Part model, mm, in its own coordinate system. Face numbers are marked on the shaded views. Coordinates: 2 decimals unless noted, no trailing zeros. Loops run counter-clockwise (first coordinate to the right, second up) from the corner with the lowest first, then second, coordinate; pieces in that order, holes last. Notation, with made-up numbers: M 70,-31.75 L 78,-31.75 A28 cw 78,-6.75 Z; hole C 33.5,61 d8. An arc over 180 degrees is marked long. Answer as a JSON object with one key per item and string values. Group by question number.
1. Drill centre lines: L1, parallel to X at y = 0, z = 7.2; L2, parallel to Y at x = 0, z = 2.1 (3 decimals); L3, parallel to X at y = -5, z = 10.5 (3 decimals). Where is each one in solid material? Low to high.
2. Drop a flat-ended pin along its axis: pin 1 Ø7.5 at (x, y) = (0, 0) entering from +Z. Give the stop position or say it passes through.
3. Mould opens along Y. For the marked faces 1, 2 and 3 say: released by +Y, released by -Y, zero draft, split by the parting line, or undercut.
4. Saw through at D-D on z = 2.25. Write the cut outline in (x, y) (3 decimals), then the cut area to 3 significant figures.
5. Saw through at C-C on z = 12. Write the cut outline in (x, y).
6. Saw through at B-B on x = 0. Write the cut outline in (y, z) (3 decimals), then the cut area to 3 significant figures.
7. Saw through at A-A on y = 0. Write the cut outline in (x, z) (3 decimals), then the cut area to 3 significant figures.
from build123d import *

# Parameters (mm, degrees)
F2_DEPTH = 25.4


with BuildPart() as f2:
    # F0 (on Front) → F2 (new body, symmetric)
    with BuildSketch(Plane.XZ):
        with BuildLine():
            Line((-19.05, 17.7), (-19.05, 0))
            Line((-19.05, 0), (19.05, 0))
            Line((19.05, 0), (19.05, 17.7))
            Line((19.05, 17.7), (12.541531, 17.7))
            ThreePointArc((12.541531, 17.7), (0, 7), (-12.541531, 17.7))
            Line((-12.541531, 17.7), (-19.05, 17.7))
        make_face()
    extrude(amount=F2_DEPTH, both=True)

    # F1 (on Front) → F3 (revolve, cut)
    with BuildSketch(Plane.XZ):
        Polygon((0, 17.176644), (-6.3, 17.176644), (-6.3, 7), (-6.3, 6.479864), (-3.275, 3), (-3.275, 0), (0, 0), align=None)
    revolve(axis=Axis((0, 0, 8.588322), (0, 0, -1)), mode=Mode.SUBTRACT)


solid = f2.part
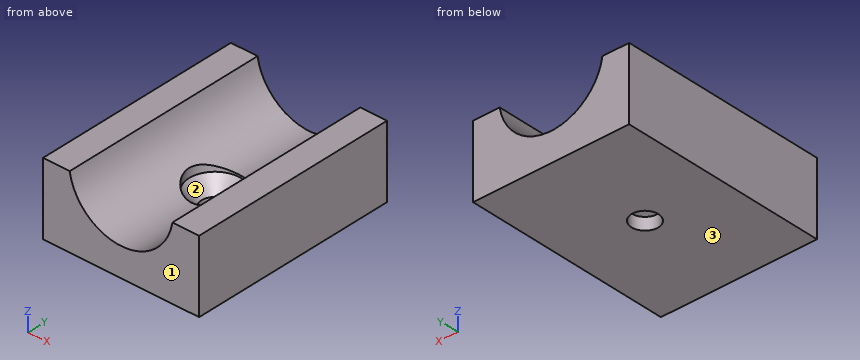
Outcome:
{
 "1": {"L1": "x = -19.05 to -6.3, 6.3 to 19.05", "L2": "y = -25.4 to -3.275, 3.275 to 25.4", "L3": "x = -19.05 to -8.755, 8.755 to 19.05"},
 "2": {"pin 1": "stops at z = 3.55"},
 "3": {"face 1": "released by -Y", "face 2": "undercut", "face 3": "zero draft"},
 "4": {"outline": "M -19.05,-25.4 L 19.05,-25.4 L 19.05,25.4 L -19.05,25.4 Z; hole C 0,0 d6.55", "area": "1,900 mm²"},
 "5": {"outline": "M -19.05,-25.4 L -10.1,-25.4 L -10.1,25.4 L -19.05,25.4 Z; M 10.1,-25.4 L 19.05,-25.4 L 19.05,25.4 L 10.1,25.4 Z"},
 "6": {"outline": "M -25.4,0 L -3.275,0 L -3.275,3 L -6.3,6.48 L -6.3,7 L -25.4,7 Z; M 3.275,0 L 25.4,0 L 25.4,7 L 6.3,7 L 6.3,6.48 L 3.275,3 Z", "area": "296 mm²"},
 "7": {"outline": "M -19.05,0 L -3.275,0 L -3.275,3 L -6.3,6.48 L -6.3,8.673 A12.7 cw -12.542,17.7 L -19.05,17.7 Z; M 3.275,0 L 19.05,0 L 19.05,17.7 L 12.542,17.7 A12.7 cw 6.3,8.673 L 6.3,6.48 L 3.275,3 Z", "area": "405 mm²"}
}
